The model under review builds one solid part; all positions refer to its coordinate system, in mm. Face numbers are marked on the shaded views. A direction names the side the tool comes from. Round coordinates to 2 decimals unless told otherwise and drop trailing zeros. Loops run counter-clockwise (first coordinate to the right, second up) from the corner with the lowest first, then second, coordinate; pieces in that order, holes last. Notation, with made-up numbers: (30.5, 4) - (64.5, 4) arc R10 ccw to (64.5, 8) - close; hole circle Ø6 at (-0.5, -12). An arc over 180 degrees is marked (long way). Answer as CSV lines item,"result".
Autodesk Inventor part; units mm, degrees
ref_plane "YZ Plane" through (0, 0, 0) normal (1, 0, 0) x (0, 1, 0)
ref_plane "XZ Plane" through (0, 0, 0) normal (0, 1, 0) x (-1, 0, 0)
ref_plane "XY Plane" through (0, 0, 0) normal (0, 0, 1) x (1, 0, 0)
sketch "Sketch1" plane through (0, 0, 0) normal (0, 0, 1) x (1, 0, 0)
  line L0 (0, 0) -> (17.5, 0)
  line L1 (17.5, 0) -> (17.5, 28)
  line L2 (17.5, 28) -> (-17.5, 28)
  line L3 (-17.5, 28) -> (-17.5, 0)
  line L4 (-17.5, 0) -> (17.5, 0)
  dimension "d0" = 17.5
  dimension "d1" = 28
  dimension "d2" = 35
extrude "Extrusion1" add sketch "Sketch1" along normal blind 30
sketch "Sketch2" plane through (0, 0, 30) normal (0, 0, 1) x (1, 0, 0)
  circle A0 centre (0, 14) radius 5.1
  line L0 (17.5, 28) -> (-17.5, 28)
  line L1 (-17.5, 28) -> (-17.5, 0)
  point P0 (0, 0)
  dimension "d5" = 10.2
  dimension "d6" = 14
  dimension "d85" = 17.5
extrude "Extrusion2" cut sketch "Sketch2" against normal blind 30
sketch "Sketch4" plane through (-17.5, 28, 0) normal (0, 1, 0) x (1, 0, 0)
  line L0 (0, -30) -> (35, -30)
  line L1 (17.5, -30) -> (17.5, 3.7121)
  line L2 (0, 0) -> (0, -30)
  circle A0 centre (29.5, -6) radius 2
  circle A1 centre (5.5, -6) radius 2
  line L3 (34, -15) -> (-3.2563, -15)
  line L4 (35, 0) -> (0, 0)
  circle A2 centre (29.5, -24) radius 2
  circle A3 centre (5.5, -24) radius 2
  line L5 (35, 0) -> (35, -30)
  dimension "d37" = 17.5
  dimension "d38" = 4
  dimension "d39" = 4
  dimension "d42" = 15
  dimension "d43" = 4
  dimension "d44" = 4
  dimension "d61" = 6
  dimension "d62" = 6
  dimension "d63" = 6
  dimension "d64" = 6
  dimension "d86" = 12
  dimension "d87" = 12
  dimension "d88" = 12
  dimension "d89" = 12
extrude "Extrusion4" cut sketch "Sketch4" against normal blind 10 contours A0 | A1 | A2 | A3
thread "Thread7"
thread "Thread8"
thread "Thread9"
thread "Thread10"
sketch "Sketch7" plane through (0, 0, 30) normal (0, 0, 1) x (1, 0, 0)
  circle A0 centre (0, 14) radius 5.1
  circle A1 centre (0, 14) radius 11
  point P0 (0, 0)
  dimension "d72" = 22
extrude "Extrusion5" cut sketch "Sketch7" against normal blind 5
sketch "Sketch9" plane through (0, 14, 25) normal (0, 0, 1) x (1, 0, 0)
  circle A0 centre (-8, 0) radius 1.5
  circle A1 centre (8, 0) radius 1.5
  point P0 (0, -14)
  dimension "d76" = 3
  dimension "d78" = 3
extrude "Extrusion6" cut sketch "Sketch9" against normal blind 10
thread "Thread11"
thread "Thread12"
properties part number "AoVitmeT8"
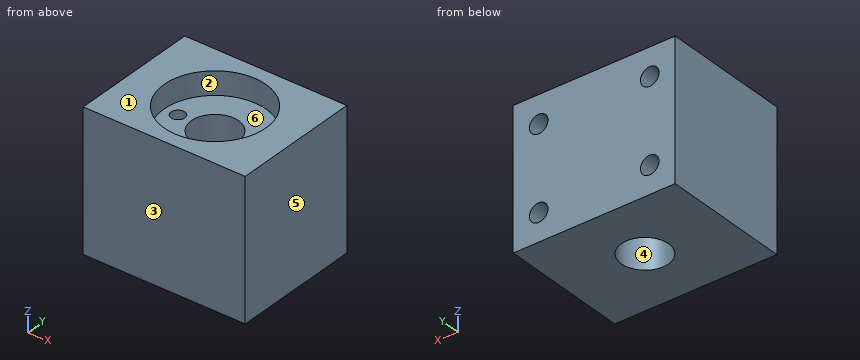
1. Take a section at B-B (z = 19.5). State the section outline as (x, y) points.
Numbers:
outline,"(-17.5, 0) - (17.5, 0) - (17.5, 28) - (-17.5, 28) - close; hole circle Ø3 at (-8, 14); hole circle Ø10.2 at (0, 14); hole circle Ø3 at (8, 14)"
2. Wall thickness on probe 1 along Z at (x, y) = (-12, 21.25); probe 2 along X at (y, z) = (24.25, 6); probe 3 along Z at (x, y) = (11, 19): over which ranges is each line inside the solid? List them lowest first.
Numbers:
probe 1,"z = 0 to 4, 8 to 22, 26 to 30"
probe 2,"x = -17.5 to -14, -10 to 10, 14 to 17.5"
probe 3,"z = 0 to 4.27, 7.73 to 22.27, 25.73 to 30"
3. Draft analysis for pull direction Y (two halves, no side actions). For the marked faces 3, 4, 5 and 6, state which applies: +Y half, -Y half, draft (parallel to the pull), parting line (faces both ways), or undercut.
Numbers:
face 3,"-Y half"
face 4,"undercut"
face 5,"draft"
face 6,"undercut"
4. Tool access review of the marked faces 1 and 2: name each direction out of +Z, -Z, +X, -X, +Y, -Y from which nothing blocks a thin tool from reaching the whole face with its end or side.
Numbers:
face 1,"+Z, +X, -X, +Y, -Y"
face 2,"+Z"
5. Take a section at C-C (x = 0). State the section outline as (y, z) points.
Numbers:
outline,"(0, 0) - (8.9, 0) - (8.9, 25) - (3, 25) - (3, 30) - (0, 30) - close; (19.1, 0) - (28, 0) - (28, 30) - (25, 30) - (25, 25) - (19.1, 25) - close"
6. Take a section at A-A (y = 14). State the section outline as (x, z) points.
Numbers:
outline,"(-17.5, 0) - (-5.1, 0) - (-5.1, 25) - (-6.5, 25) - (-6.5, 15) - (-9.5, 15) - (-9.5, 25) - (-11, 25) - (-11, 30) - (-17.5, 30) - close; (5.1, 0) - (17.5, 0) - (17.5, 30) - (11, 30) - (11, 25) - (9.5, 25) - (9.5, 15) - (6.5, 15) - (6.5, 25) - (5.1, 25) - close"
7. Take a section at D-D (z = 6). State the section outline as (x, y) points.
Numbers:
outline,"(-17.5, 0) - (17.5, 0) - (17.5, 28) - (14, 28) - (14, 18) - (10, 18) - (10, 28) - (-10, 28) - (-10, 18) - (-14, 18) - (-14, 28) - (-17.5, 28) - close; hole circle Ø10.2 at (0, 14)"
8. Clearance check with flat-ended pins moving along their axes: pin 1 (2 mm diameter, centred on x = 0, y = 8.5, fed in from +Z); pin 2 (1.2 mm diameter, centred on x = 12.5, z = 5.5, fed in from +Y); pin 3 (6 mm diameter, centred on x = -7, y = 20, fed in from +Z); pin 4 (1.5 mm diameter, centred on x = -7.5, y = 13.5, fed in from +Z). State where each tip first meets the part, or that it passes through.
Numbers:
pin 1,"stops at z = 25"
pin 2,"stops at y = 18"
pin 3,"stops at z = 30"
pin 4,"stops at z = 15"
